Model file for the job. Use its own axes, mm. A direction names the side the tool comes from. Round coordinates to 2 decimals unless told otherwise and drop trailing zeros. Order: outer loops, then holes, each group sorted by start corner. A loop starts at its lowest first (then second) coordinate and runs counter-clockwise, first axis right, second up. Notation, with made-up numbers: (-32.75, 77.5) -> (21.25, 77.5) arc R18 cw to (21.25, 104.5) -> close; hole circle Ø4 at (57, -1). An arc over 180 degrees is marked (long way). Answer as CSV lines item,"result".
```python
from build123d import *

# Parameters (mm, degrees)
FLAT_PLATE_W       = 98.425
FLAT_PLATE_H       = 114.3
CASTOR_PLATE_DEPTH = 3.175
CUT_EXTRUDE1_DEPTH = 3.175


with BuildPart() as part:
    # Flat Plate → Castor Plate (new body)
    with BuildSketch(Plane.XY):
        with Locations((-52.168585316, -18.955051946)):
            Rectangle(FLAT_PLATE_W, FLAT_PLATE_H)
    extrude(amount=CASTOR_PLATE_DEPTH)

    # Holes → Cut-Extrude1 (cut)
    with BuildSketch(Plane.XY.offset(3.175)):
        with BuildLine():
            Line((-96.801649102, 16.159330585), (-84.977633144, 29.437924132))
            ThreePointArc((-84.977633144, 29.437924132), (-76.012415463, 29.957416129), (-75.492923466, 20.992198448))
            Line((-75.492923466, 20.992198448), (-87.316939425, 7.7136049))
            ThreePointArc((-87.316939425, 7.7136049), (-96.282157106, 7.194112904), (-96.801649102, 16.159330585))
        make_face()
        with BuildLine():
            Line((-29.762145467, -60.410465456), (-17.938129508, -47.131871908))
            ThreePointArc((-17.938129508, -47.131871908), (-8.972911827, -46.612379911), (-8.453419831, -55.577597592))
            Line((-8.453419831, -55.577597592), (-20.27743579, -68.85619114))
            ThreePointArc((-20.27743579, -68.85619114), (-29.242653471, -69.375683136), (-29.762145467, -60.410465456))
        make_face()
        with BuildLine():
            Line((-88.615669415, -46.990896649), (-75.337075868, -58.814912608))
            ThreePointArc((-75.337075868, -58.814912608), (-74.817583871, -67.780130289), (-83.782801552, -68.299622285))
            Line((-83.782801552, -68.299622285), (-97.0613951, -56.475606326))
            ThreePointArc((-97.0613951, -56.475606326), (-97.580887096, -47.510388645), (-88.615669415, -46.990896649))
        make_face()
        with BuildLine():
            Line((-21.57616578, 30.126649102), (-8.297572232, 18.302633144))
            ThreePointArc((-8.297572232, 18.302633144), (-7.778080236, 9.337415463), (-16.743297917, 8.817923466))
            Line((-16.743297917, 8.817923466), (-30.021891465, 20.641939425))
            ThreePointArc((-30.021891465, 20.641939425), (-30.541383461, 29.607157106), (-21.57616578, 30.126649102))
        make_face()
    extrude(amount=-CUT_EXTRUDE1_DEPTH, mode=Mode.SUBTRACT)


solid = part.part
```
Q1. Saw through at C-C (z = 0.95). Write the cut outline in (x, y).
Checks:
outline,"(-101.38, -76.11) -> (-2.96, -76.11) -> (-2.96, 38.19) -> (-101.38, 38.19) -> close; hole (-97.06, -56.48) -> (-83.78, -68.3) arc R6.35 ccw to (-75.34, -58.81) -> (-88.62, -46.99) arc R6.35 ccw to start; hole (-96.8, 16.16) arc R6.35 ccw to (-87.32, 7.71) -> (-75.49, 20.99) arc R6.35 ccw to (-84.98, 29.44) -> close; hole (-30.02, 20.64) -> (-16.74, 8.82) arc R6.35 ccw to (-8.3, 18.3) -> (-21.58, 30.13) arc R6.35 ccw to start; hole (-29.76, -60.41) arc R6.35 ccw to (-20.28, -68.86) -> (-8.45, -55.58) arc R6.35 ccw to (-17.94, -47.13) -> close"
Q2. Tool access for faces 4 (the flat face through (-15.03, 24.3, 1.61)), 5 (the flat face through (-53, -18, 3.175)): list every direction of +Z, -Z, +X, -X, +Y, -Y with a clear straight run to the whole face (end or side of a thin tool).
Checks:
face 4,"+Z, -Z"
face 5,"+Z, +X, -X, +Y, -Y"
Q3. Mould opens along X. For faces 1 (the flat face through (-82.07, -52.82, 1.61)), 2 (the flat face through (-101.381, -20, 2)), 3 (the flat face through (-2.956, -20, 2)) say: +X half, -X half, draft (parallel to the pull), parting line (faces both ways), or undercut.
Checks:
face 1,"undercut"
face 2,"-X half"
face 3,"+X half"
Q4. Wall check: L1, parallel to X at y = 17.5, z = 0.55; L2, parallel to Y at x = -29, z = 2.55; L3, parallel to Y at x = -8.5, z = 1.6. Give the ranges that are in metal, low to high. Write a range as [from, to].
Checks:
L1,"[-101.38, -95.61], [-78.6, -26.49], [-7.54, -2.96]"
L2,"[-76.11, -69.58], [-59.55, 19.73], [30.87, 38.19]"
L3,"[-76.11, -55.63], [-47.08, 8.65], [18.48, 38.19]"
Q5. Saw through at A-A (x = -24). Write the cut outline in (y, z) (3 decimals).
Checks:
outline,"(-76.105, 0) -> (-70.901, 0) -> (-70.901, 3.175) -> (-76.105, 3.175) -> close; (-53.939, 0) -> (15.28, 0) -> (15.28, 3.175) -> (-53.939, 3.175) -> close; (31.474, 0) -> (38.195, 0) -> (38.195, 3.175) -> (31.474, 3.175) -> close"
Q6. Saw through at B-B (y = 25). Write the cut outline in (x, z) (3 decimals), plus the area to 3 significant figures.
Checks:
outline,"(-101.381, 0) -> (-88.929, 0) -> (-88.929, 3.175) -> (-101.381, 3.175) -> close; (-73.889, 0) -> (-32.137, 0) -> (-32.137, 3.175) -> (-73.889, 3.175) -> close; (-15.819, 0) -> (-2.956, 0) -> (-2.956, 3.175) -> (-15.819, 3.175) -> close"
area,"213 mm²"
